Job drawing, mm, ordinate dimensions from the low corner. One solid piece. A direction names the side the tool comes from. Round coordinates to 2 decimals unless told otherwise and drop trailing zeros. Order: outer loops, then holes, each group sorted by start corner. A loop starts at its lowest first (then second) coordinate and runs counter-clockwise, first axis right, second up. Notation, with made-up numbers: (-10.5, 20) -> (13.5, 20) arc R19 ccw to (13.5, 56) -> close; hole circle Ø3 at (-34.5, 46). An arc over 180 degrees is marked (long way). Return JSON: item names as keys, results as strings. Group by question number.
Q1. Mould opens along Z. For the marked faces 5, 6, 7 and 8 say: +Z half, -Z half, draft (parallel to the pull), parting line (faces both ways), or undercut.
Q2. Probe line 1 along Y through (x, z) = (53, 23); line 2 along Y through (x, z) = (39.5, 45.5); line 3 along Z through (x, y) = (61, 86). List the from-to ranges inside material, lowest first.
Q3. Flat gauge pins, fed straight in: pin 1 (8.5 mm diameter, centred on x = 45.5, z = 15.5, fed in from -Y); pin 2 (5 mm diameter, centred on y = 78, z = 11.5, fed in from -X); pin 3 (20 mm diameter, centred on y = 42, z = 23, fed in from -X); pin 4 (3 mm diameter, centred on y = 47.5, z = 2.5, fed in from +X). Where does each tip first touch, or does it go through?
Q4. Cut at A-A (z = 50). Write the cut outline in (x, y), then the cut area to 3 significant figures.
Q5. Which spindle directions (+Z, -Z, +X, -X, +Y, -Y) get a long thin tool onto all of the face, cutting with end or side? Do the marked faces 1, 2, 3 and 4. Say none if no direction does.
Q6. Cut at D-D (x = 67). Write the cut outline in (y, z), then the cut area to 3 significant figures.
Q7. Cut at C-C (y = 42). Write the cut outline in (x, z) (1 decimal).
Q8. Cut at B-B (x = 54). Write the cut outline in (y, z) (1 decimal).
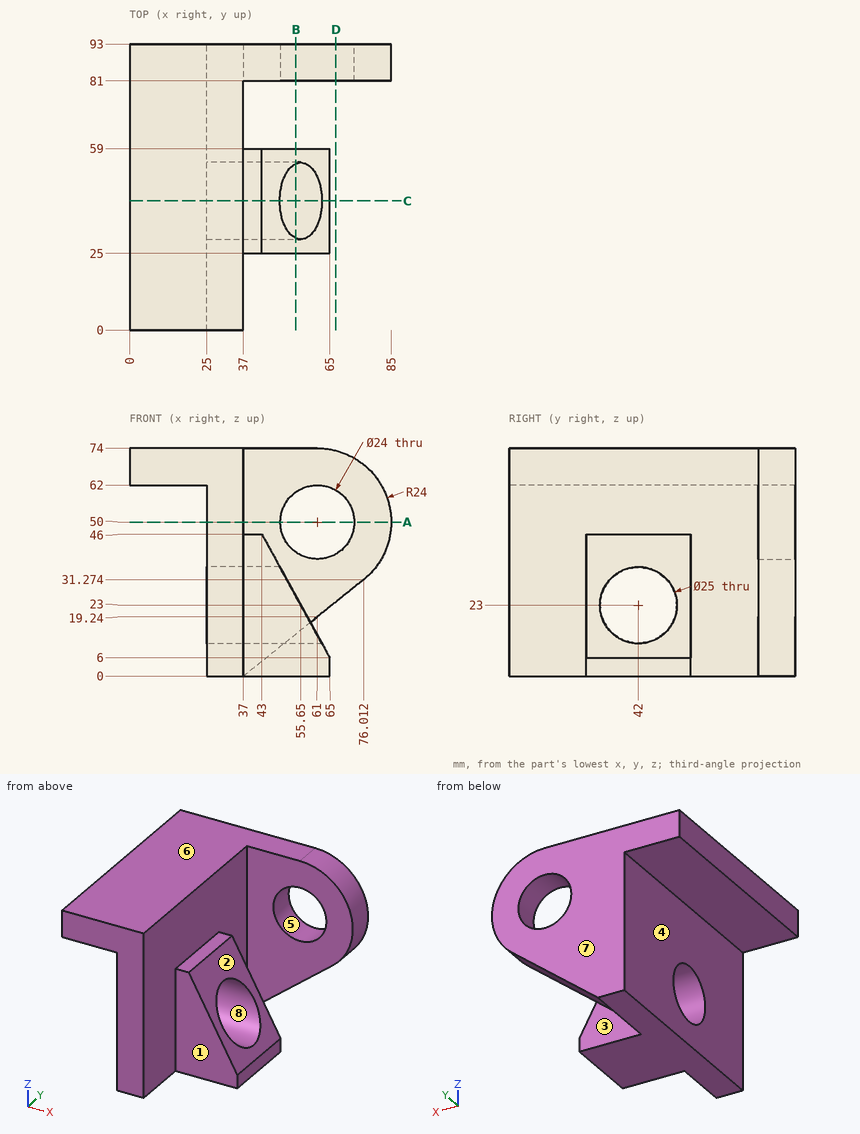
Solution:
{
 "1": {"face 5": "undercut", "face 6": "+Z half", "face 7": "draft", "face 8": "undercut"},
 "2": {"line 1": "y = 25 to 29.5, 54.5 to 59, 81 to 93", "line 2": "y = 25 to 59, 81 to 93", "line 3": "z = 19.24 to 38, 62 to 74"},
 "3": {"pin 1": "stops at y = 25", "pin 2": "stops at x = 25", "pin 3": "passes through", "pin 4": "stops at x = 65"},
 "4": {"outline": "(25, 0) -> (37, 0) -> (37, 81) -> (49, 81) -> (49, 93) -> (25, 93) -> close; (73, 81) -> (85, 81) -> (85, 93) -> (73, 93) -> close", "area": "1,400 mm²"},
 "5": {"face 1": "+Z, -Z, +X, -Y", "face 2": "+Z, +X, -Y", "face 3": "+Z, -Z, +X", "face 4": "-Z, -X, +Y, -Y"},
 "6": {"outline": "(81, 24.05) -> (93, 24.05) -> (93, 39.61) -> (81, 39.61) -> close; (81, 60.39) -> (93, 60.39) -> (93, 73.24) -> (81, 73.24) -> close", "area": "341 mm²"},
 "7": {"outline": "(0, 62) -> (25, 62) -> (25, 35.5) -> (48.8, 35.5) -> (43, 46) -> (37, 46) -> (37, 74) -> (0, 74) -> close; (25, 0) -> (65, 0) -> (65, 6) -> (62.5, 10.5) -> (25, 10.5) -> close"},
 "8": {"outline": "(25, 0) -> (59, 0) -> (59, 26) -> (54.1, 26) arc R12.5 cw (long way) to (29.9, 26) -> (25, 26) -> close; (81, 13.6) -> (93, 13.6) -> (93, 40.3) -> (81, 40.3) -> close; (81, 59.7) -> (93, 59.7) -> (93, 74) -> (81, 74) -> close"}
}
